Geometry: final body of the model. Coordinates: model frame, mm. Coordinates: 2 decimals unless noted, no trailing zeros. Loops run counter-clockwise (first coordinate to the right, second up) from the corner with the lowest first, then second, coordinate; pieces in that order, holes last. Notation, with made-up numbers: (60, 1) -> (82, 1) arc R19 cw to (82, 29) -> close; hole circle Ø8 at (89.25, 38). An arc over 180 degrees is marked (long way). One line per item, written item: value. Start each with the question number.
Item 1: Section query C-C on z = -5.75. Give the number of separate pieces and of enclosed holes in the cut face, then the cut area to 3 significant figures.
Item 2: Contact query for flat-ended pins moving along their axis: pin 1 Ø3 at (y, z) = (-29, -2.5) entering from +X; pin 2 Ø1 at (y, z) = (4, -1.5) entering from +X; pin 3 Ø3 at (y, z) = (-19, -7) entering from -X. Output: stop coordinate, or through.
Item 3: Section query A-A on y = -28. Return loops of the section in (x, z), then the cut area to 3 significant figures.
Item 4: Section query B-B on x = -7. Return loops of the section in (y, z).
Item 5: Section query D-D on y = -21. Return loops of the section in (x, z), then the cut area to 3 significant figures.
Item 6: Ray query, probe 1 along Y at (x, z) = (-9, -5); probe 2 along Y at (x, z) = (0, -7.5); probe 3 along Y at (x, z) = (-13, -6.75). Return the intervals inside material, ascending. Write a range as from..to.
Item 7: Mould query, pull axis Y, two halves, no side actions, for faces 1 (the flat face through (11.2, -21.6, -5.7)), 2 (the cylindrical face through (-8.96, 0.85, -5.67)), 3 (the flat face through (-5, -1, 0)). Classes: +Y half, -Y half, draft (parallel to the pull), parting line (faces both ways), or undercut.
Autodesk Inventor part; units mm, degrees
ref_plane "YZ Plane" through (0, 0, 0) normal (1, 0, 0) x (0, 1, 0)
ref_plane "XZ Plane" through (0, 0, 0) normal (0, 1, 0) x (-1, 0, 0)
ref_plane "XY Plane" through (0, 0, 0) normal (0, 0, 1) x (1, 0, 0)
ref_plane "РабПлоскость1" through (0, 0, 0) normal (0, 0, 1) x (1, 0, 0)
sketch "Эскиз1" plane through (0, 0, 0) normal (0, 0, 1) x (1, 0, 0)
  circle A0 centre (0, 0) radius 15
  circle A1 centre (-9.5, 0) radius 1.0064
  circle A2 centre (0, -12.5) radius 1.0064
  circle A3 centre (0, 12.5) radius 1.0064
  circle A4 centre (9.5, 0) radius 1.0064
  circle A5 centre (0, 0) radius 2
  circle A6 centre (0, 0) radius 2.15
  circle A7 centre (-16.5815, 12.0542) radius 3
  circle A8 centre (-10.1413, -32.4523) radius 8.075
  circle A9 centre (-19.85, 6.2031) radius 2.5 construction
  circle A10 centre (-5, -16) radius 2.5 construction
  circle A11 centre (19.85, -6.2031) radius 2.5 construction
  line L0 (19.85, -6.2031) -> (-19.85, 6.2031) construction
  line L1 (-10.1413, -32.4523) -> (-5, -16) construction
  circle A12 centre (-10.1413, -32.4523) radius 4 construction
  circle A13 centre (-10.1413, -32.4523) radius 12.5 construction
  circle A14 centre (-10.1413, -32.4523) radius 10
  line L2 (-0.5965, -35.4351) -> (-19.6861, -29.4696) construction
  circle A15 centre (0, 0) radius 24.5
  circle A16 centre (-16.5815, 12.0542) radius 4 construction
  line L3 (-0.5965, -35.4351) -> (23.3848, -7.3077)
  line L4 (-19.6861, -29.4696) -> (-23.3848, 7.3077)
  point P0 (-19.6861, -29.4696)
  dimension "d9" = 20
  dimension "d0" = 4.3
  dimension "d1" = 6
  dimension "d2" = 16.15
  dimension "d3" = 5
  dimension "d4" = 5
  dimension "d5" = 5
  dimension "d6" = 8
  dimension "d7" = 25
  dimension "d8" = 34
  dimension "d10" = 8
  dimension "d11" = 49
extrude "Выдавливание1" add sketch "Эскиз1" against normal blind 11.5 contours A0 | A14 A15 | L4 A15 A14 | A14 A15 L3 | A15 L4 L3 A14 | A14 A15
properties part number "DriblerWall"
Reply:
1. separate pieces: 1
1. enclosed holes: 7
1. area: 2,010 mm²
2. pin 1: stops at x = 6.17
2. pin 2: stops at x = 24.25
2. pin 3: stops at x = -20.89
3. outline: (-19.83, -11.5) -> (-16.88, -11.5) -> (-16.88, 0) -> (-19.83, 0) -> close; (-3.4, -11.5) -> (5.74, -11.5) -> (5.74, 0) -> (-3.4, 0) -> close
3. area: 139 mm²
4. outline: (-41.95, -11.5) -> (-39.89, -11.5) -> (-39.89, 0) -> (-41.95, 0) -> close; (-25.01, -11.5) -> (23.48, -11.5) -> (23.48, 0) -> (-25.01, 0) -> close
5. outline: (-20.54, -11.5) -> (11.71, -11.5) -> (11.71, 0) -> (-20.54, 0) -> close
5. area: 371 mm²
6. probe 1: y = -42.39..-40.45, -24.46..-0.87, 0.87..22.79
6. probe 2: y = -34.74..-13.51, -11.49..-2.15, 2.15..11.49, 13.51..24.5
6. probe 3: y = -42.03..-40, -24.9..20.77
7. face 1: -Y half
7. face 2: undercut
7. face 3: draft
